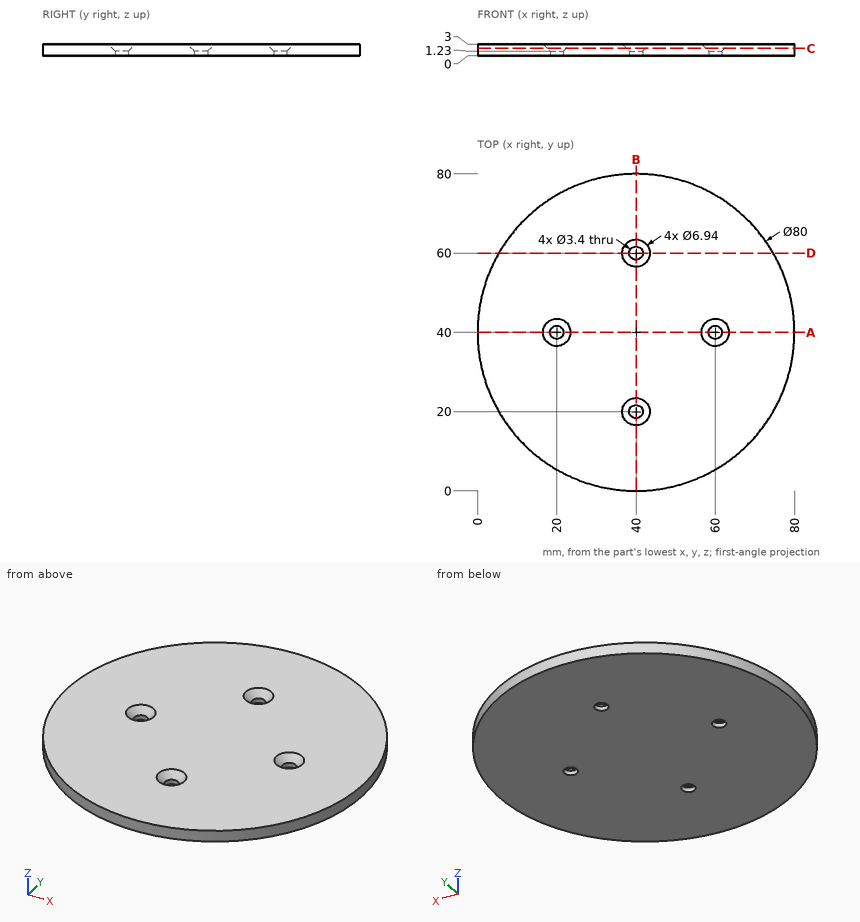
Check sheet for the drawn part. Datum: minimum x, y, z corner. Units: mm. Round coordinates to 2 decimals unless told otherwise and drop trailing zeros. Order: outer loops, then holes, each group sorted by start corner. A loop starts at its lowest first (then second) coordinate and runs counter-clockwise, first axis right, second up. Notation, with made-up numbers: (13, 51.5) - (66, 51.5) arc R3 ccw to (66, 56.5) - close; hole circle Ø5 at (73.5, 48.25). An arc over 180 degrees is marked (long way). Use a Markdown table: item, result. Add a question column.
(1) Sectioned sample at C-C, the plane z = 1.9. Enter the section's corners in (x, y).
(2) Depth check by flat-ended pin: pin 1 (3 mm diameter, centred on x = 40, y = 20, fed in from -Z); pin 2 (4.5 mm diameter, centred on x = 40, y = 60, fed in from +Z); pin 3 (5.5 mm diameter, centred on x = 60, y = 40, fed in from +Z). Enter the tip coordinate at first touch or a pass-through.
(3) Sectioned sample at D-D, the plane y = 60. Enter the section's corners in (x, z), and give its area (3 significant figures).
(4) Sectioned sample at A-A, the plane y = 40. Enter the section's corners in (x, z), and give its area (3 significant figures).
(5) Material ranges on line 1 along Y through (x, z) = (40, 0.4); line 2 along Y through (x, z) = (20, 0.35); line 3 along Y through (x, z) = (61.5, 2), recorded low to high. Write a range as [from, to].
Answers below:
| question | item | result |
|---|---|---|
| 1 | outline | circle Ø80 at (40, 40); hole circle Ø4.74 at (20, 40); hole circle Ø4.74 at (40, 20); hole circle Ø4.74 at (40, 60); hole circle Ø4.74 at (60, 40) |
| 2 | pin 1 | through |
| 2 | pin 2 | z = 1.78 |
| 2 | pin 3 | z = 2.28 |
| 3 | outline | (5.36, 0) - (38.3, 0) - (38.3, 1.23) - (36.53, 3) - (5.36, 3) - close; (41.7, 0) - (74.64, 0) - (74.64, 3) - (43.47, 3) - (41.7, 1.23) - close |
| 3 | area | 195 mm² |
| 4 | outline | (0, 0) - (18.3, 0) - (18.3, 1.23) - (16.53, 3) - (0, 3) - close; (21.7, 0) - (58.3, 0) - (58.3, 1.23) - (56.53, 3) - (23.47, 3) - (21.7, 1.23) - close; (61.7, 0) - (80, 0) - (80, 3) - (63.47, 3) - (61.7, 1.23) - close |
| 4 | area | 213 mm² |
| 5 | line 1 | [0, 18.3], [21.7, 58.3], [61.7, 80] |
| 5 | line 2 | [5.36, 38.3], [41.7, 74.64] |
| 5 | line 3 | [6.27, 38.04], [41.96, 73.73] |
